```python
from build123d import *

# Parameters (mm, degrees)
BOSS_EXTRUDE1_DEPTH      = 1.6
CHAMFER1_SIZE            = 2
SKETCH2_W                = 12
SKETCH2_H                = 16.6
BOSS_EXTRUDE2_DEPTH      = 10.65
SKETCH3_W                = 2.4
SKETCH3_H                = 15.6
SKETCH3_H_2              = 20.7
BOSS_EXTRUDE3_DEPTH      = 8.7
BOSS_EXTRUDE4_DEPTH      = 1.75
BOSS_EXTRUDE4_DEPTH_BACK = 1.5
SKETCH4_W                = 9
SKETCH4_H                = 11
SKETCH5_W                = 9
SKETCH5_H                = 10.5
BOSS_EXTRUDE5_DEPTH      = 10.5
FILLET1_R                = 4.5


with BuildPart() as part:
    # Sketch1 → Boss-Extrude1 (new body)
    with BuildSketch(Plane(origin=(0, 0, 0), x_dir=(1, 0, 0), z_dir=(0, 1, 0))):
        Polygon((-26.75, -66), (-23.75, -66), (-20.75, -69), (10.75, -69), (13.75, -66), (26.75, -66), (26.75, 0), (-26.75, 0), align=None)
    extrude(amount=BOSS_EXTRUDE1_DEPTH)

    # Chamfer1
    chamfer1_edges = [part.edges().sort_by_distance(p)[0] for p in [
        (26.75, 0.8, 66),
    ]]
    chamfer(chamfer1_edges, length=CHAMFER1_SIZE)

    # Sketch2 → Boss-Extrude2 (add)
    with BuildSketch(Plane(origin=(0, 1.6, 0), x_dir=(1, 0, 0), z_dir=(0, 1, 0))):
        with Locations((11.25, -1.8)):
            Rectangle(SKETCH2_W, SKETCH2_H)
    extrude(amount=BOSS_EXTRUDE2_DEPTH)

    # Sketch3 → Boss-Extrude3 (add)
    with BuildSketch(Plane(origin=(0, 1.6, 0), x_dir=(1, 0, 0), z_dir=(0, 1, 0))):
        with Locations((-24.05, -56.7)):
            Rectangle(SKETCH3_W, SKETCH3_H)
        with Locations((-24.05, -39.1)):
            Rectangle(SKETCH3_W, SKETCH3_H)
        with Locations((24.05, -54.15)):
            Rectangle(SKETCH3_W, SKETCH3_H_2)
        with Locations((24.05, -32.45)):
            Rectangle(SKETCH3_W, SKETCH3_H_2)
    extrude(amount=BOSS_EXTRUDE3_DEPTH)

    # Sketch4 → Boss-Extrude4 (add, two sides: drawn at the far end of the back side and taken through both)
    with BuildSketch(Plane(origin=(0, 0, 0), x_dir=(-1, 0, 0), z_dir=(0, 0, -1)).offset(-BOSS_EXTRUDE4_DEPTH_BACK)):
        with Locations((18.75, 7.1)):
            Rectangle(SKETCH4_W, SKETCH4_H)
    extrude(amount=BOSS_EXTRUDE4_DEPTH + BOSS_EXTRUDE4_DEPTH_BACK)

    # Sketch5 → Boss-Extrude5 (add)
    with BuildSketch(Plane.XY.offset(1.5)):
        with Locations((-18.75, 6.85)):
            Rectangle(SKETCH5_W, SKETCH5_H)
    extrude(amount=BOSS_EXTRUDE5_DEPTH)

    # Fillet1
    fillet1_edges = [part.edges().sort_by_distance(p)[0] for p in [
        (-14.25, 12.1, 6.75),
        (-23.25, 12.1, 6.75),
    ]]
    fillet(fillet1_edges, radius=FILLET1_R - 0.0001)  # a hair under: the kernel refuses the full size


solid = part.part
```
CAD build for the part. Positions are in the model's coordinates, mm. A direction names the side the tool comes from. Round coordinates to 2 decimals unless told otherwise and drop trailing zeros. Loops run counter-clockwise (first coordinate to the right, second up) from the corner with the lowest first, then second, coordinate; pieces in that order, holes last. Notation, with made-up numbers: (-37.75, -14) - (20.25, -14) arc R16 cw to (20.25, 13) - close; hole circle Ø8 at (-38.75, 30.5). An arc over 180 degrees is marked (long way). Return JSON: item names as keys, results as strings. Group by question number.
Q1. Tool access for faces 4 (the face through (25.25, 6, 33)), 5 (the face through (-23.25, 6, 4)), 6 (the face through (24, 6, 22.1)), 7 (the face through (-15.533, 10.747, 6.824)): list every direction of +Z, -Z, +X, -X, +Y, -Y with a clear straight run to the whole face (end or side of a thin tool).
Q2. Drill centre lines: line 1 along X through (y, z) = (8, 32); line 2 along Y through (x, z) = (-5, 53.5); line 3 along Z through (x, y) = (7.5, 5.75). Where is each one in solid material? Low to high. Write a range as [from, to].
Q3. Band-saw the part on A-A on y = 3.75. Give the cut face in (x, z).
Q4. Band-saw the part on C-C on z = 33. Give the cut face in (x, y).
Q5. Flat gauge pins, fed straight in: pin 1 Ø0.5 at (x, y) = (13, 0.5) entering from -Z; pin 2 Ø3 at (x, y) = (18, 5) entering from +Z; pin 3 Ø1.2 at (x, y) = (23.5, 4) entering from +Z; pin 4 Ø8 at (x, z) = (-3, 20.5) entering from -Y. Where does each tip first touch, or does it go through?
Q6. Band-saw the part on B-B on x = 8. Give the cut face in (y, z).
Q7. Band-saw the part on D-D on y = 8.75. Give the cut face in (x, z), plus the area to 3 significant figures.
Q8. Two-plate mould, pull along Z, no slides. Class faces 1 (the face through (-21.967, 10.747, 6.824)), 2 (the face through (11, 7, -6.5)), 3 (the face through (22.85, 6, 33)): +Z half, -Z half, draft (parallel to the pull), parting line (faces both ways), or undercut.
Solutions:
{
 "1": {"face 4": "+Z, -Z, +X, +Y", "face 5": "-Z, -X, +Y", "face 6": "-Z, +X, -X, +Y", "face 7": "+Z, +Y"},
 "2": {"line 1": "x = [-25.25, -22.85], [22.85, 25.25]", "line 2": "y = [0, 1.6]", "line 3": "z = [-6.5, 10.1]"},
 "3": {"outline": "(-25.25, 31.3) - (-22.85, 31.3) - (-22.85, 46.9) - (-25.25, 46.9) - close; (-25.25, 48.9) - (-22.85, 48.9) - (-22.85, 64.5) - (-25.25, 64.5) - close; (-23.25, -1.75) - (-14.25, -1.75) - (-14.25, 12) - (-23.25, 12) - close; (5.25, -6.5) - (17.25, -6.5) - (17.25, 10.1) - (5.25, 10.1) - close; (22.85, 22.1) - (25.25, 22.1) - (25.25, 42.8) - (22.85, 42.8) - close; (22.85, 43.8) - (25.25, 43.8) - (25.25, 64.5) - (22.85, 64.5) - close"},
 "4": {"outline": "(-26.75, 0) - (26.75, 0) - (26.75, 1.6) - (25.25, 1.6) - (25.25, 10.3) - (22.85, 10.3) - (22.85, 1.6) - (-22.85, 1.6) - (-22.85, 10.3) - (-25.25, 10.3) - (-25.25, 1.6) - (-26.75, 1.6) - close"},
 "5": {"pin 1": "stops at z = 0", "pin 2": "stops at z = 10.1", "pin 3": "stops at z = 64.5", "pin 4": "stops at y = 0"},
 "6": {"outline": "(0, 0) - (1.6, 0) - (1.6, -6.5) - (12.25, -6.5) - (12.25, 10.1) - (1.6, 10.1) - (1.6, 69) - (0, 69) - close"},
 "7": {"outline": "(-25.25, 31.3) - (-22.85, 31.3) - (-22.85, 46.9) - (-25.25, 46.9) - close; (-25.25, 48.9) - (-22.85, 48.9) - (-22.85, 64.5) - (-25.25, 64.5) - close; (-23.25, -1.75) - (-14.25, -1.75) - (-14.25, 1.5) - (-14.4, 1.5) - (-14.4, 12) - (-23.1, 12) - (-23.1, 1.5) - (-23.25, 1.5) - close; (5.25, -6.5) - (17.25, -6.5) - (17.25, 10.1) - (5.25, 10.1) - close; (22.85, 22.1) - (25.25, 22.1) - (25.25, 42.8) - (22.85, 42.8) - close; (22.85, 43.8) - (25.25, 43.8) - (25.25, 64.5) - (22.85, 64.5) - close", "area": "494 mm^2"},
 "8": {"face 1": "undercut", "face 2": "-Z half", "face 3": "draft"}
}
